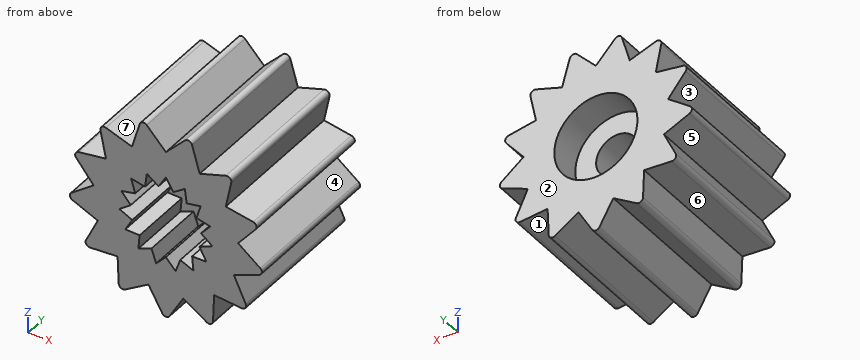
from build123d import *

# Parameters (mm, degrees)
SKETCH1_R           = 1
BOSS_EXTRUDE1_DEPTH = 7
CUT_EXTRUDE1_DEPTH  = 3
FILLET1_R           = 0.2
SKETCH3_R           = 2
CUT_EXTRUDE2_DEPTH  = 1.5


with BuildPart() as part:
    # Sketch1 → Boss-Extrude1 (new body)
    with BuildSketch(Plane(origin=(0, 0, 0), x_dir=(1, 0, 0), z_dir=(0, 1, 0))):
        Polygon((2.320929304, 2.619787619), (3.990706765, 2.754585991), (3.272556849, 1.241117105), (4.813715291, 0.584490857), (3.474481059, -0.421878381), (4.533959656, -1.719504088), (2.880443531, -1.988226614), (3.215528503, -3.629581369), (1.626531102, -3.09909609), (1.160458522, -4.708165299), (0, -3.5), (-1.160458522, -4.708165299), (-1.626531102, -3.09909609), (-3.215528503, -3.629581369), (-2.880443531, -1.988226614), (-4.533959656, -1.719504088), (-3.474481059, -0.421878381), (-4.813715291, 0.584490857), (-3.272556849, 1.241117105), (-3.990706765, 2.754585991), (-2.320929304, 2.619787619), (-2.253475412, 4.293638671), (-0.837604825, 3.398296361), (0, 4.849070475), (0.837604825, 3.398296361), (2.253475412, 4.293638671), align=None)
        with Locations(Location((0, 0, 0), (0, 0, 270))):
            Circle(SKETCH1_R, mode=Mode.SUBTRACT)
    extrude(amount=BOSS_EXTRUDE1_DEPTH)

    # Sketch2 → Cut-Extrude1 (cut)
    with BuildSketch(Plane.XZ):
        Polygon((0, 2.25), (-0.353449874, 1.662850921), (-0.915157447, 2.05547728), (-0.999234929, 1.37532889), (-1.672075857, 1.505543864), (-1.472243186, 0.85), (-2.139877162, 0.695288237), (-1.690687222, 0.177698388), (-2.237674265, -0.235189042), (-1.616796078, -0.52532889), (-1.948557159, -1.125), (-1.263346203, -1.137522031), (-1.322516818, -1.820288237), (-0.691452293, -1.553027278), (-0.467801304, -2.200832102), (0, -1.7), (0.467801304, -2.200832102), (0.691452293, -1.553027278), (1.322516818, -1.820288237), (1.263346203, -1.137522031), (1.948557159, -1.125), (1.616796078, -0.52532889), (2.237674265, -0.235189042), (1.690687222, 0.177698388), (2.139877162, 0.695288237), (1.472243186, 0.85), (1.672075857, 1.505543864), (0.999234929, 1.37532889), (0.915157447, 2.05547728), (0.353449874, 1.662850921), align=None)
    extrude(amount=-CUT_EXTRUDE1_DEPTH, mode=Mode.SUBTRACT)

    # Fillet1
    fillet1_edges = [part.edges().sort_by_distance(p)[0] for p in [
        (4.813715291, 3.5, -0.584490857),
        (4.533959656, 3.5, 1.719504088),
        (3.215528503, 3.5, 3.629581369),
        (1.160458522, 3.5, 4.708165299),
        (-1.160458522, 3.5, 4.708165299),
        (-3.215528503, 3.5, 3.629581369),
        (-4.533959656, 3.5, 1.719504088),
        (-4.813715291, 3.5, -0.584490857),
        (-3.990706765, 3.5, -2.754585991),
        (-2.253475412, 3.5, -4.293638671),
        (0, 3.5, -4.849070475),
        (2.253475412, 3.5, -4.293638671),
        (3.990706765, 3.5, -2.754585991),
    ]]
    fillet(fillet1_edges, radius=FILLET1_R)

    # Sketch3 → Cut-Extrude2 (cut)
    with BuildSketch(Plane(origin=(0, 7, 0), x_dir=(1, 0, 0), z_dir=(0, 1, 0))):
        with Locations(Location((0, 0, 0), (0, 0, 270))):
            Circle(SKETCH3_R)
    extrude(amount=-CUT_EXTRUDE2_DEPTH, mode=Mode.SUBTRACT)


solid = part.part
Can you work these out from the model? Positions are in its coordinate system, mm. Face numbers are marked on the shaded views. A direction names the side the tool comes from. Coordinates: 2 decimals unless noted, no trailing zeros. Write each loop counter-clockwise with the first axis right and the second up, starting at its lowest first coordinate (ties: lowest second). Pieces come first, ordered by that corner, then holes. Notation, with made-up numbers: (69, 1.25) -> (92, 1.25) arc R5 ccw to (92, 8.25) -> close; hole circle Ø9 at (-1, 31.25). An arc over 180 degrees is marked (long way). Write item = value, one per line.
(1) If I drill on probe 1 along Y at (x, z) = (-0.5, 1.25); probe 2 along X at (y, z) = (3.8, 0); probe 3 along X at (y, z) = (6.75, -3.75), over which ranges is the centre line in solid material (lowest first)?
Verdict:
probe_1 = 3 to 5.5
probe_2 = -4.04 to -1, 1 to 4.04
probe_3 = -2.28 to -1.39, -0.63 to 0.63, 1.39 to 2.28
(2) Imagine slicing it at A-A (z = 0). Please give me the cut outline in (x, y), and give its area (3 significant figures).
Verdict:
outline = (-4.04, 0) -> (-1.93, 0) -> (-1.93, 3) -> (-1, 3) -> (-1, 5.5) -> (-2, 5.5) -> (-2, 7) -> (-4.04, 7) -> close; (1, 3) -> (1.93, 3) -> (1.93, 0) -> (4.04, 0) -> (4.04, 7) -> (2, 7) -> (2, 5.5) -> (1, 5.5) -> close
area = 33.9 mm^2
(3) On a 3-axis mill with a long thin cutter (end or side, diameter ignored), from which of +Z, -Z, +X, -X, +Y, -Y can I reach the whole of each face in a straight line? I mean the marked faces 5, 6 and 7. Say none if no direction works.
Verdict:
face_5 = -X, +Y, -Y
face_6 = -Z, +Y, -Y
face_7 = +Z, +Y, -Y
(4) Imagine slicing it at B-B (z = -3.25). Please give me the cut outline in (x, y).
Verdict:
outline = (-2.3, 0) -> (2.3, 0) -> (2.3, 7) -> (-2.3, 7) -> close
(5) Thinking about a two-plate mould opening in X: for the marked faces 1, 2, 3 and 4, which applies, +X half, -X half, draft (parallel to the pull), parting line (faces both ways), or undercut?
Verdict:
face_1 = undercut
face_2 = draft
face_3 = -X half
face_4 = +X half
(6) For pin 1 (1.3 mm diameter, centred on x = 0.5, z = 0.5, fed in from -Y); pin 2 (1 mm diameter, centred on x = -3.5, y = 2.5, fed in from +Z); pin 3 (2.5 mm diameter, centred on x = 0, z = 0, fed in from +Y), each with a flat end and sliding along its axis, tell me the tip position at first contact or that it passes through.
Verdict:
pin_1 = 3
pin_2 = 3.52
pin_3 = 5.5
